from build123d import *

# Parameters (mm, degrees)
EXTRUDE_1_DEPTH     = 3
SKETCH_2_R          = 2.1
SKETCH_2_R_2        = 1.6
CUT_EXTRUDE_1_DEPTH = 67.211781429


with BuildPart() as part:
    # 草图1 → 凸台-拉伸1 (new body)
    with BuildSketch(Plane.XY):
        Polygon((0, 0), (-30, 0), (-30, 50), (0, 50), (17.057713659, 32.942286341), (33.301270189, 42.320508076), (43.301270189, 25), align=None)
    extrude(amount=EXTRUDE_1_DEPTH)

    # 草图2 → 切除-拉伸1 (cut, through all)
    with BuildSketch(Plane.XY.offset(3)):
        with Locations((-23, 43)):
            Circle(SKETCH_2_R)
        with Locations((-7, 43)):
            Circle(SKETCH_2_R)
        with Locations((-23, 7)):
            Circle(SKETCH_2_R)
        with Locations((-7, 7)):
            Circle(SKETCH_2_R)
        with Locations((-23, 25)):
            Circle(SKETCH_2_R)
        with Locations((-7, 25)):
            Circle(SKETCH_2_R)
        with Locations((30.605117767, 34.990381057)):
            Circle(SKETCH_2_R_2)
        with Locations((35.605117767, 26.330127019)):
            Circle(SKETCH_2_R_2)
        with Locations((22.61473671, 18.830127019)):
            Circle(SKETCH_2_R_2)
        with Locations((17.61473671, 27.490381057)):
            Circle(SKETCH_2_R_2)
        with Locations((4.624355653, 19.990381057)):
            Circle(SKETCH_2_R_2)
        with Locations((9.624355653, 11.330127019)):
            Circle(SKETCH_2_R_2)
    extrude(amount=-CUT_EXTRUDE_1_DEPTH, mode=Mode.SUBTRACT)


solid = part.part
Can you work these out from the model? Positions are in its coordinate system, mm. A direction names the side the tool comes from. Give positions to 0.01 mm unless a question says otherwise; leave off trailing zeros. Order: outer loops, then holes, each group sorted by start corner. A loop starts at its lowest first (then second) coordinate and runs counter-clockwise, first axis right, second up. Notation, with made-up numbers: M 32.25,6.25 L 85.25,6.25 A22 cw 85.25,39.25 Z; hole C -17,65 d2. An arc over 180 degrees is marked long. Use a Markdown table: item, result. Add a question column.
Item 1: Will this pin go through, and if not, where does the flat tip stop? pin 1 (1.5 mm diameter, centred on x = 19.5, z = 1.5, fed in from +Y).
Item 2: Suppose I cut it at C-C (x = 26). List the corners of the cut face in (y, z) for me.
Item 3: If I drill on L1, parallel to X at y = 42.5, z = 2.7; L2, parallel to X at y = 19, z = 1.7; L3, parallel to X at y = 40.5, z = 2.8, over which ranges is the centre line in solid material (lowest first)? Write a range as [from, to].
Item 4: For faces 1 (the flat face through (25.07, 37.57, 1.48)), 2 (the cylindrical face through (-8.548, 26.419, 1.521)), which set-ups out of +Z, -Z, +X, -X, +Y, -Y let a thin tool reach every point of the face, with its end or its side?
Item 5: Suppose I cut it at A-A (x = -23). List the corners of the cut face in (y, z) for me.
Item 6: Suppose I cut it at B-B (z = 1.6). Count the separate pieces of the cut face and the enclosed holes in it, then the cut area to 3 significant figures.
Item 7: We'd pull the mould along Y, two halves only. Please class faces 3 (the cylindrical face through (4.278, 18.428, 1.521)), 4 (the flat face through (-15, 50, 1)), 5 (the cylindrical face through (17.406, 29.077, 1.521)), 6 (the flat face through (-1, 25, 0)): +Y half, -Y half, draft (parallel to the pull), parting line (faces both ways), or undercut.
Answer sheet:
| question | item | result |
|---|---|---|
| 1 | pin 1 | stops at y = 34.79 |
| 2 | outline | M 15.01,0 L 38.11,0 L 38.11,3 L 15.01,3 Z |
| 3 | L1 | x = [-30, -25.04], [-20.96, -9.04], [-4.96, 7.5] |
| 3 | L2 | x = [-30, 3.37], [5.88, 21.02], [24.21, 32.91] |
| 3 | L3 | x = [-30, 9.5], [30.15, 34.35] |
| 4 | face 1 | +Z, -Z, +Y |
| 4 | face 2 | +Z, -Z |
| 5 | outline | M 0,0 L 4.9,0 L 4.9,3 L 0,3 Z; M 9.1,0 L 22.9,0 L 22.9,3 L 9.1,3 Z; M 27.1,0 L 40.9,0 L 40.9,3 L 27.1,3 Z; M 45.1,0 L 50,0 L 50,3 L 45.1,3 Z |
| 6 | separate pieces | 1 |
| 6 | enclosed holes | 12 |
| 6 | area | 2,480 mm² |
| 7 | face 3 | undercut |
| 7 | face 4 | +Y half |
| 7 | face 5 | undercut |
| 7 | face 6 | draft |
